from build123d import *

# Parameters (mm, degrees)
F1_DEPTH     = 22
F2_DEPTH     = 3
F3_DEPTH     = 15
F0_W         = 15
F0_H         = 30
F4_DEPTH     = 15
F5_R         = 2
F6_T1_DEPTH  = 111.1292207426
F6_T3_DEPTH  = 68.4264144678
F6_T5_DEPTH  = 14.1054111362
F6_T10_DEPTH = 2
F6_T14_ANGLE = 24.9330990778
F7_R         = 1
F8_R         = 1
F9_DEPTH     = 5


# Not quite as in the source:
# - a fillet or chamfer that OpenCascade refuses, or shapes differently, is made with other operations: its cross-section is extruded or revolved along the edge and cut away or added
# - a feature names something its author has since deleted; it is built from what else it names


with BuildPart() as f1:
    # F0 (on Top) → F1 (new body)
    with BuildSketch(Plane.XY):
        with BuildLine():
            ThreePointArc((93, 77.5), (92.267766953, 79.267766953), (90.5, 80))
            Line((90.5, 80), (36.5, 80))
            Line((36.5, 80), (24.5, 80))
            Line((24.5, 80), (19, 80))
            Line((19, 80), (-7, 80))
            Line((-7, 80), (-12.5, 80))
            Line((-12.5, 80), (-24.5, 80))
            Line((-24.5, 80), (-74, 80))
            Line((-74, 80), (-91.5, 80))
            ThreePointArc((-91.5, 80), (-93.267766953, 79.267766953), (-94, 77.5))
            Line((-94, 77.5), (-94, 76))
            Line((-94, 76), (-94, 0))
            Line((-94, 0), (-94, -1.5))
            ThreePointArc((-94, -1.5), (-93.267766953, -3.267766953), (-91.5, -4))
            Line((-91.5, -4), (-88, -4))
            Line((-88, -4), (-73, -4))
            Line((-73, -4), (-28.6959191337, -4))
            Line((-28.6959191337, -4), (67.7072161436, -4))
            Line((67.7072161436, -4), (88, -3.7670015892))
            Line((88, -3.7670015892), (90.5, -3.7670015892))
            ThreePointArc((90.5, -3.7670015892), (92.267766953, -3.0347685421), (93, -1.2670015892))
            Line((93, -1.2670015892), (93, 0))
            Line((93, 0), (93, 76))
            Line((93, 76), (93, 77.5))
        make_face()
        with BuildLine():
            ThreePointArc((90, 2.5), (89.267766953, 0.732233047), (87.5, 0))
            Line((87.5, 0), (-87.5, 0))
            ThreePointArc((-87.5, 0), (-89.267766953, 0.732233047), (-90, 2.5))
            Line((-90, 2.5), (-90, 73.5))
            ThreePointArc((-90, 73.5), (-89.267766953, 75.267766953), (-87.5, 76))
            Line((-87.5, 76), (87.5, 76))
            ThreePointArc((87.5, 76), (89.267766953, 75.267766953), (90, 73.5))
            Line((90, 73.5), (90, 2.5))
        make_face(mode=Mode.SUBTRACT)
    extrude(amount=F1_DEPTH)

    # F0 (on Top) → F2 (join)
    with BuildSketch(Plane.XY):
        with BuildLine():
            Line((-87.5, 0), (87.5, 0))
            ThreePointArc((87.5, 0), (89.267766953, 0.732233047), (90, 2.5))
            Line((90, 2.5), (90, 73.5))
            ThreePointArc((90, 73.5), (89.267766953, 75.267766953), (87.5, 76))
            Line((87.5, 76), (-87.5, 76))
            ThreePointArc((-87.5, 76), (-89.267766953, 75.267766953), (-90, 73.5))
            Line((-90, 73.5), (-90, 2.5))
            ThreePointArc((-90, 2.5), (-89.267766953, 0.732233047), (-87.5, 0))
        make_face()
        with BuildLine():
            Line((-77.5, 66), (77.5, 66))
            ThreePointArc((77.5, 66), (79.267766953, 65.267766953), (80, 63.5))
            Line((80, 63.5), (80, 12.5))
            ThreePointArc((80, 12.5), (79.267766953, 10.732233047), (77.5, 10))
            Line((77.5, 10), (-77.5, 10))
            ThreePointArc((-77.5, 10), (-79.267766953, 10.732233047), (-80, 12.5))
            Line((-80, 12.5), (-80, 63.5))
            ThreePointArc((-80, 63.5), (-79.267766953, 65.267766953), (-77.5, 66))
        make_face(mode=Mode.SUBTRACT)
    extrude(amount=F2_DEPTH)

    # F0 (on Top) → F3 (join)
    with BuildSketch(Plane.XY):
        with BuildLine():
            Line((93, -81.2670015892), (93, -1.2670015892))
            ThreePointArc((93, -1.2670015892), (92.267766953, -3.0347685421), (90.5, -3.7670015892))
            Line((90.5, -3.7670015892), (88, -3.7670015892))
            Line((88, -3.7670015892), (67.7072161436, -4))
            ThreePointArc((67.7072161436, -4), (74.7782839555, -6.9289321881), (77.7072161436, -14))
            Line((77.7072161436, -14), (77.7072161436, -58.7379819401))
            ThreePointArc((77.7072161436, -58.7379819401), (73.0879609173, -67.1669549309), (63.4976990076, -67.8088124137))
            Line((63.4976990076, -67.8088124137), (-32.9054362697, -23.0708304737))
            ThreePointArc((-32.9054362697, -23.0708304737), (-38.4608642113, -11.8445771571), (-28.6959191337, -4))
            Line((-28.6959191337, -4), (-73, -4))
            Line((-73, -4), (-73, -34))
            Line((-73, -34), (-24.5735855322, -34))
            ThreePointArc((-24.5735855322, -34), (-24.033911544, -34.0589444934), (-23.5196862036, -34.2329984108))
            Line((-23.5196862036, -34.2329984108), (77.653316815, -81.2670015892))
            Line((77.653316815, -81.2670015892), (93, -81.2670015892))
        make_face()
    extrude(amount=F3_DEPTH)

    # F0 (on Top) → F4 (join)
    with BuildSketch(Plane.XY):
        with Locations((-80.5, -19)):
            Rectangle(F0_W, F0_H)
    extrude(amount=F4_DEPTH)

    # F5
    f5_edges = [f1.edges().sort_by_distance(p)[0] for p in [
        (85.326658, -81.267002, 15),
    ]]
    fillet(f5_edges, radius=F5_R)

    # F6: fillet of radius 2 on 4 edges, made by hand

    # F6_s2 → F6_t1 (cut)
    with BuildSketch(Plane(origin=(-6.2536714965, 2.9072499211, 0), x_dir=(0, 0, 1), z_dir=(0.9068006357, -0.4215597314, 0))):
        with BuildLine():
            ThreePointArc((15, 38.9574573188), (14.4142135624, 40.3716708812), (13, 40.9574573188))
            Line((13, 40.9574573188), (15, 40.9574573188))
            Line((15, 40.9574573188), (15, 38.9574573188))
        make_face()
    extrude(amount=F6_T1_DEPTH, mode=Mode.SUBTRACT)

    # F6_s4 → F6_t3 (cut)
    with BuildSketch(Plane.YZ.offset(-93)):
        with BuildLine():
            ThreePointArc((-32, 15), (-33.4142135624, 14.4142135624), (-34, 13))
            Line((-34, 13), (-34, 15))
            Line((-34, 15), (-32, 15))
        make_face()
    extrude(amount=F6_T3_DEPTH, mode=Mode.SUBTRACT)

    # F6_s6 → F6_t5 (cut)
    with BuildSketch(Plane.XY.offset(-1.1054111362)):
        with BuildLine():
            ThreePointArc((77.2523618067, -81.0806028605), (77.6637420789, -81.2198459945), (78.0954812695, -81.2670015892))
            Line((78.0954812695, -81.2670015892), (77.653316815, -81.2670015892))
            Line((77.653316815, -81.2670015892), (77.2523618067, -81.0806028605))
        make_face()
    extrude(amount=F6_T5_DEPTH, mode=Mode.SUBTRACT)


with BuildPart() as f6_tool8:
    # F6_s9 → F6_t10 (new body)
    with BuildSketch(Plane.XY.offset(13)):
        Polygon((78.0954812695, -79.2670015892), (78.0954812695, -81.2670015892), (77.653316815, -81.2670015892), (77.2523618067, -81.0806028605), align=None)
    extrude(amount=F6_T10_DEPTH)

    # F6_s11 → F6_t12 (revolve, cut)
    with BuildSketch(Plane(origin=(78.0954812695, -79.2670015892, 13), x_dir=(0.2158695953, 0.9764222027, 0), z_dir=(0.9764222027, -0.2158695953, 0))):
        with BuildLine():
            ThreePointArc((0, -2), (2, 0), (0, 2))
            Line((0, 2), (0, -2))
        make_face()
    revolve(axis=Axis((78.0954812695, -79.2670015892, 13), (0, 0, 1)), mode=Mode.SUBTRACT)


with BuildPart() as f1_1:
    add(f1.part)

    # F6_t7: cut F6_tool8
    add(f6_tool8.part, mode=Mode.SUBTRACT)

    # F6_s13 → F6_t14 (revolve, cut)
    with BuildSketch(Plane.YZ.offset(-24.5735855322)):
        with BuildLine():
            ThreePointArc((-32, 15), (-33.4142135624, 14.4142135624), (-34, 13))
            Line((-34, 13), (-34, 15))
            Line((-34, 15), (-32, 15))
        make_face()
    revolve(axis=Axis((-24.5735855322, -36.5, 15), (0, 0, -1)), revolution_arc=F6_T14_ANGLE, mode=Mode.SUBTRACT)

    # F7
    f7_edges = [f1_1.edges().sort_by_distance(p)[0] for p in [
        (93, -81.267002, 6.5),
    ]]
    fillet(f7_edges, radius=F7_R)

    # F8
    f8_edges = [f1_1.edges().sort_by_distance(p)[0] for p in [
        (-88, -34, 6.5),
        (-88, -18, 15),
        (-88, -33.414214, 14.414214),
    ]]
    fillet(f8_edges, radius=F8_R)

    # F0 (on Top) → F9 (join)
    with BuildSketch(Plane.XY):
        with BuildLine():
            Line((-24.5, 80), (-12.5, 80))
            Line((-12.5, 80), (-12.5, 89.5))
            ThreePointArc((-12.5, 89.5), (-13.232233047, 91.267766953), (-15, 92))
            Line((-15, 92), (-22, 92))
            ThreePointArc((-22, 92), (-23.767766953, 91.267766953), (-24.5, 89.5))
            Line((-24.5, 89.5), (-24.5, 80))
        make_face()
        with BuildLine():
            Line((-7, 80), (19, 80))
            Line((19, 80), (19, 89.5))
            ThreePointArc((19, 89.5), (18.267766953, 91.267766953), (16.5, 92))
            Line((16.5, 92), (-4.5, 92))
            ThreePointArc((-4.5, 92), (-6.267766953, 91.267766953), (-7, 89.5))
            Line((-7, 89.5), (-7, 80))
        make_face()
        with BuildLine():
            Line((24.5, 80), (36.5, 80))
            Line((36.5, 80), (36.5, 89.5))
            ThreePointArc((36.5, 89.5), (35.767766953, 91.267766953), (34, 92))
            Line((34, 92), (27, 92))
            ThreePointArc((27, 92), (25.232233047, 91.267766953), (24.5, 89.5))
            Line((24.5, 89.5), (24.5, 80))
        make_face()
    extrude(amount=F9_DEPTH)


solid = f1_1.part
Here's how the part is built. I have some questions about the finished solid (model axes, mm). A direction names the side the tool comes from. Give positions to 0.01 mm unless a question says otherwise; leave off trailing zeros. Loops run counter-clockwise (first coordinate to the right, second up) from the corner with the lowest first, then second, coordinate; pieces in that order, holes last. Notation, with made-up numbers: (-12.75, 18) -> (32.25, 18) arc R19 ccw to (32.25, 41) -> close; hole circle Ø2 at (-1.5, -29). An arc over 180 degrees is marked (long way). Answer as a JSON object with one key per item and string values. Group by question number.
Item 1: Will these pins go through, and if not, where does the flat tip stop? pin 1 (2 mm diameter, centred on x = 89.5, z = 18.5, fed in from -Y); pin 2 (2 mm diameter, centred on x = 20, z = 18, fed in from -Y); pin 3 (11 mm diameter, centred on x = -49, z = 14.5, fed in from -Y).
Item 2: Imagine slicing it at A-A on y = 50.5. Write out the boundary of the cut face in (x, z), then the cut area to 3 significant figures.
Item 3: On a 3-axis mill with a long thin cutter (end or side, diameter ignored), from which of +Z, -Z, +X, -X, +Y, -Y can I reach the whole of each face in a straight line? I mean faces 1 (the flat face through (1, 0, 12)), 2 (the flat face through (-56, -34, 6)), 3 (the flat face through (15.971, -45.753, 7.395)), 4 (the flat face through (-24.5, 85, 2)), 5 (the flat face through (24.5, 85, 2)). Say none if no direction works.
Item 4: Thinking about a two-plate mould opening in Y: for faces 6 (the flat face through (6, 86, 5)), 7 (the cylindrical face through (73.21, -67.09, 7.4)), 8 (the flat face through (26.16, -57.33, 6.41)), 9 (the flat face through (-0.4, 66.3, 3)), which applies, pulls with the +Y half, pulls with the -Y half, needs draft (parallel to the pull), parting line crosses it, or undercut?
Item 5: Imagine slicing it at B-B on z = 9.25. Give the number of separate pieces and of enclosed holes in the cut face, then the cut area to 3 significant figures.
Item 6: I need wall thicknesses on L1, parallel to X at y = 80.5, z = 2.5; L2, parallel to Y at x = 73.5, z = 13.5; L3, parallel to X at y = 54.5, z = 17.25. Which ranges of each line are inside material? Lowest first, please.
Item 7: Imagine slicing it at D-D on y = -27. Write out the boundary of the cut face in (x, z).
Answer list:
{
 "1": {"pin 1": "stops at y = -3.77", "pin 2": "stops at y = -4", "pin 3": "stops at y = -34"},
 "2": {"outline": "(-94, 0) -> (-80, 0) -> (-80, 3) -> (-90, 3) -> (-90, 22) -> (-94, 22) -> close; (80, 0) -> (93, 0) -> (93, 22) -> (90, 22) -> (90, 3) -> (80, 3) -> close", "area": "214 mm2"},
 "3": {"face 1": "+Z", "face 2": "+Z, -Z, -X, -Y", "face 3": "+Z, -Z", "face 4": "+Z, -Z, -X, +Y", "face 5": "+Z, -Z, +Y"},
 "4": {"face 6": "needs draft", "face 7": "undercut", "face 8": "pulls with the -Y half", "face 9": "undercut"},
 "5": {"separate pieces": "1", "enclosed holes": "2", "area": "5,640 mm2"},
 "6": {"L1": "x = -24.5 to -12.5, -7 to 19, 24.5 to 36.5", "L2": "y = -79.27 to -66.89, -5.85 to 0, 76 to 80", "L3": "x = -94 to -90, 90 to 93"},
 "7": {"outline": "(-88, 0) -> (-24.44, 0) -> (-24.44, 15) -> (-87, 15) arc R1 ccw to (-88, 14) -> close; (77.71, 0) -> (93, 0) -> (93, 14) arc R1 ccw to (92, 15) -> (77.71, 15) -> close"}
}
